from build123d import *

# Parameters (mm, degrees)
SKETCH_1_R          = 6
EXTRUDE_1_DEPTH     = 1.5
EXTRUDE_2_DEPTH     = 3
SKETCH_6_R          = 0.6
CUT_EXTRUDE_2_DEPTH = 4
FILLET_1_R          = 1.5
SKETCH_7_R          = 1.55
CUT_EXTRUDE_3_DEPTH = 4
CUT_EXTRUDE_4_DEPTH = 4
FILLET_2_R          = 0.6
SKETCH_9_W          = 1.5
SKETCH_9_H          = 1.5
EXTRUDE_3_DEPTH     = 3
SKETCH_10_R         = 0.6
CUT_EXTRUDE_5_DEPTH = 4


with BuildPart() as part:
    # 草图1 → 凸台-拉伸1 (new body, symmetric)
    with BuildSketch(Plane.XY):
        with BuildLine():
            Line((-12.5, 12), (12.5, 12))
            Line((12.5, 12), (19.728184266, -3.500891181))
            Line((19.728184266, -3.500891181), (30.763838853, -7.517540966))
            ThreePointArc((30.763838853, -7.517540966), (40.374225454, -4.092068476), (38.803964436, 5.988986664))
            Line((38.803964436, 5.988986664), (27.5, 16))
            Line((27.5, 16), (-27.5, 16))
            Line((-27.5, 16), (-38.803964436, 5.988986664))
            ThreePointArc((-38.803964436, 5.988986664), (-40.374225454, -4.092068476), (-30.763838853, -7.517540966))
            Line((-30.763838853, -7.517540966), (-19.728184266, -3.500891181))
            Line((-19.728184266, -3.500891181), (-12.5, 12))
        make_face()
        with Locations((-33.5, 0)):
            Circle(SKETCH_1_R, mode=Mode.SUBTRACT)
        with Locations((33.5, 0)):
            Circle(SKETCH_1_R, mode=Mode.SUBTRACT)
    extrude(amount=EXTRUDE_1_DEPTH, both=True)

    # 草图5 → 凸台-拉伸2 (add)
    with BuildSketch(Plane.XY.offset(1.5)):
        Polygon((-14.001000824, 8.781093345), (-9.922615783, 6.879311167), (-14.1487984, -2.183766703), (-18.227183442, -0.281984526), (-17.170637787, 1.983784942), (-14.90486832, 0.927239288), (-12.791777011, 5.458778223), (-15.057546479, 6.515323877), align=None)
        Polygon((14.90486832, 0.927239288), (17.170637787, 1.983784942), (18.227183442, -0.281984526), (14.1487984, -2.183766703), (9.922615783, 6.879311167), (14.001000824, 8.781093345), (15.057546479, 6.515323877), (12.791777011, 5.458778223), align=None)
    extrude(amount=-EXTRUDE_2_DEPTH)

    # 草图6 → 切除-拉伸2 (cut, through all)
    with BuildSketch(Plane.XY.offset(1.5)):
        with Locations((-15.311117436, 5.971539205)):
            Circle(SKETCH_6_R)
        with Locations((-13.045347968, 4.914993551)):
            Circle(SKETCH_6_R)
        with Locations((-16.91706683, 2.527569614)):
            Circle(SKETCH_6_R)
        with Locations((-14.651297363, 1.47102396)):
            Circle(SKETCH_6_R)
        with Locations((-13.747429867, 9.324878017)):
            Circle(SKETCH_6_R)
        with Locations((-18.480754399, -0.825769198)):
            Circle(SKETCH_6_R)
        with Locations((18.480754399, -0.825769198)):
            Circle(SKETCH_6_R)
        with Locations((13.747429867, 9.324878017)):
            Circle(SKETCH_6_R)
        with Locations((14.651297363, 1.47102396)):
            Circle(SKETCH_6_R)
        with Locations((16.91706683, 2.527569614)):
            Circle(SKETCH_6_R)
        with Locations((13.045347968, 4.914993551)):
            Circle(SKETCH_6_R)
        with Locations((15.311117436, 5.971539205)):
            Circle(SKETCH_6_R)
        with Locations((-11.956215328, 11.746429043)):
            Circle(SKETCH_6_R)
        with Locations((11.956215328, 11.746429043)):
            Circle(SKETCH_6_R)
    extrude(amount=-CUT_EXTRUDE_2_DEPTH, mode=Mode.SUBTRACT)

    # 圆角1
    fillet_1_edges = [part.edges().sort_by_distance(p)[0] for p in [
        (-9.922615783, 6.879311167, 0),
        (-14.1487984, -2.183766703, 0),
        (14.1487984, -2.183766703, 0),
        (9.922615783, 6.879311167, 0),
    ]]
    fillet(fillet_1_edges, radius=FILLET_1_R)

    # 草图7 → 切除-拉伸3 (cut, through all)
    with BuildSketch(Plane.XY.offset(1.5)):
        with Locations((-22.24449722, -0.615436184)):
            Circle(SKETCH_7_R)
        with Locations((-16.327841555, 12.072872835)):
            Circle(SKETCH_7_R)
        with Locations((22.24449722, -0.615436184)):
            Circle(SKETCH_7_R)
        with Locations((16.327841555, 12.072872835)):
            Circle(SKETCH_7_R)
    extrude(amount=-CUT_EXTRUDE_3_DEPTH, mode=Mode.SUBTRACT)

    # 草图8 → 切除-拉伸4 (cut, through all)
    with BuildSketch(Plane.XY.offset(1.5)):
        with BuildLine():
            Line((-26.172964956, 12.5), (-31.531802084, 7.754108393))
            ThreePointArc((-31.531802084, 7.754108393), (-29.20884675, 6.751740797), (-27.315064556, 5.074108154))
            Line((-27.315064556, 5.074108154), (-23.85231432, 12.5))
            Line((-23.85231432, 12.5), (-26.172964956, 12.5))
        make_face()
        with BuildLine():
            Line((-22.101342595, 5.607063857), (-21.002535115, 7.963464103))
            ThreePointArc((-21.002535115, 7.963464103), (-20.205179486, 8.253677818), (-20.495393201, 9.051033448))
            Line((-20.495393201, 9.051033448), (-22.761162668, 10.107579102))
            ThreePointArc((-22.761162668, 10.107579102), (-23.558518298, 9.817365387), (-23.268304582, 9.020009758))
            Line((-23.268304582, 9.020009758), (-24.367112063, 6.663609511))
            ThreePointArc((-24.367112063, 6.663609511), (-25.164467692, 6.373395796), (-24.874253977, 5.576040167))
            Line((-24.874253977, 5.576040167), (-22.608484509, 4.519494512))
            ThreePointArc((-22.608484509, 4.519494512), (-21.81112888, 4.809708228), (-22.101342595, 5.607063857))
        make_face()
        with BuildLine():
            Line((24.874253977, 5.576040167), (22.608484509, 4.519494512))
            ThreePointArc((22.608484509, 4.519494512), (21.81112888, 4.809708228), (22.101342595, 5.607063857))
            Line((22.101342595, 5.607063857), (21.002535115, 7.963464103))
            ThreePointArc((21.002535115, 7.963464103), (20.205179486, 8.253677818), (20.495393201, 9.051033448))
            Line((20.495393201, 9.051033448), (22.761162668, 10.107579102))
            ThreePointArc((22.761162668, 10.107579102), (23.558518298, 9.817365387), (23.268304582, 9.020009758))
            Line((23.268304582, 9.020009758), (24.367112063, 6.663609511))
            ThreePointArc((24.367112063, 6.663609511), (25.164467692, 6.373395796), (24.874253977, 5.576040167))
        make_face()
        with BuildLine():
            Line((26.172964956, 12.5), (23.85231432, 12.5))
            Line((23.85231432, 12.5), (27.315064556, 5.074108154))
            ThreePointArc((27.315064556, 5.074108154), (29.20884675, 6.751740797), (31.531802084, 7.754108393))
            Line((31.531802084, 7.754108393), (26.172964956, 12.5))
        make_face()
    extrude(amount=-CUT_EXTRUDE_4_DEPTH, mode=Mode.SUBTRACT)

    # 圆角2
    fillet_2_edges = [part.edges().sort_by_distance(p)[0] for p in [
        (26.172964956, 12.5, 0),
        (31.531802084, 7.754108393, 0),
        (27.315064556, 5.074108154, 0),
        (23.85231432, 12.5, 0),
        (-26.172964956, 12.5, 0),
        (-23.85231432, 12.5, 0),
        (-27.315064556, 5.074108154, 0),
        (-31.531802084, 7.754108393, 0),
    ]]
    fillet(fillet_2_edges, radius=FILLET_2_R)

    # 草图9 → 凸台-拉伸3 (add)
    with BuildSketch(Plane.XY.offset(1.5)):
        with Locations((0, 16.75)):
            Rectangle(SKETCH_9_W, SKETCH_9_H)
    extrude(amount=-EXTRUDE_3_DEPTH)

    # 草图10 → 切除-拉伸5 (cut, through all)
    with BuildSketch(Plane.XY.offset(1.5)):
        with Locations((1.35, 16)):
            Circle(SKETCH_10_R)
        with Locations((-1.35, 16)):
            Circle(SKETCH_10_R)
    extrude(amount=-CUT_EXTRUDE_5_DEPTH, mode=Mode.SUBTRACT)


solid = part.part
Can you work these out from the model? Positions are in its coordinate system, mm. A direction names the side the tool comes from. Give positions to 0.01 mm unless a question says otherwise; leave off trailing zeros. Order: outer loops, then holes, each group sorted by start corner. A loop starts at its lowest first (then second) coordinate and runs counter-clockwise, first axis right, second up. Notation, with made-up numbers: M -33,40 L -14,40 A16 cw -14,68 Z; hole C 59.5,53.5 d9. An arc over 180 degrees is marked long. Use one line per item in the form item = value.
Item 1: For faces 4 (the flat face through (-16.849, -0.925, 0.021)), 5 (the flat face through (16.106, 4.266, 0.021)), 6 (the flat face through (-0.2, 12.4, -1.5)), which set-ups out of +Z, -Z, +X, -X, +Y, -Y let a thin tool reach every point of the face, with its end or its side?
Values follow:
face_4 = +Z, -Z, -Y
face_5 = +Z, -Z
face_6 = -Z, +X, -X, +Y, -Y
Item 2: If we section it at B-B, the plane z = 0.35: Count the separate pieces of the cut face and the enclosed holes in it, and give its area (3 significant figures).
Values follow:
separate_pieces = 1
enclosed_holes = 12
area = 778 mm^2
Item 3: If I drill on line 1 along Y through (x, z) = (17, 1.2); line 2 along X through (y, z) = (1.25, -0.2); line 3 along X through (y, z) = (0.5, 0.8), over which ranges is the centre line in solid material (lowest first)? Write a range as [from, to].
Values follow:
line_1 = [-0.85, 1.9], [3.12, 10.68], [13.47, 16]
line_2 = [-41.4, -39.37], [-27.63, -15.6], [-14.09, -12.55], [12.55, 14.09], [15.6, 27.63], [39.37, 41.4]
line_3 = [-41.48, -39.48], [-27.52, -23.32], [-21.17, -12.9], [12.9, 21.17], [23.32, 27.52], [39.48, 41.48]
Item 4: If we section it at A-A, the plane x = 33.5: Write out the boundary of the cut face in (y, z), and give its area (3 significant figures).
Values follow:
outline = M -8,-1.5 L -6,-1.5 L -6,1.5 L -8,1.5 Z; M 6,-1.5 L 10.69,-1.5 L 10.69,1.5 L 6,1.5 Z
area = 20.1 mm^2
Item 5: Thinking about a two-plate mould opening in Y: for faces 1 (the flat face through (-23.81, 7.86, 0.02)), 2 (the flat face through (15, 16, 0)), 3 (the cylindrical face through (-14.346, -1.594, -0.021)), which applies, pulls with the +Y half, pulls with the -Y half, needs draft (parallel to the pull), parting line crosses it, or undercut?
Values follow:
face_1 = undercut
face_2 = pulls with the +Y half
face_3 = pulls with the -Y half
Item 6: Will these pins go through, and if not, where does the flat tip stop? pin 1 Ø1 at (y, z) = (4.5, 0) entering from +X; pin 2 Ø1.5 at (y, z) = (2.5, -0.5) entering from -X; pin 3 Ø0.6 at (x, z) = (25.5, 0) entering from -Y.
Values follow:
pin_1 = 40.43
pin_2 = -41.31
pin_3 = -5.71
